The listing builds one solid part. Answer for the finished solid, in the listing's coordinates (mm). A direction names the side the tool comes from. Give positions to 0.01 mm unless a question says otherwise; leave off trailing zeros. Loops run counter-clockwise (first coordinate to the right, second up) from the corner with the lowest first, then second, coordinate; pieces in that order, holes last. Notation, with made-up numbers: M -18.5,14.5 L 7.5,14.5 A23 cw 7.5,53.5 Z; hole C 18.5,-29 d6. An arc over 180 degrees is marked long. Return JSON: item names as keys, results as strings.
from build123d import *

# Parameters (mm, degrees)
F0_W     = 45.36
F0_H     = 15
F0_R     = 1.85
F1_DEPTH = 8
F3_DEPTH = 25
F5_DEPTH = 100


with BuildPart() as f1:
    # F0 (on Top) → F1 (new body)
    with BuildSketch(Plane.XY):
        with BuildLine():
            ThreePointArc((27.5, -14), (17.600505, -9.899495), (13.5, 0))
            ThreePointArc((13.5, 0), (0, 13.5), (-13.5, 0))
            ThreePointArc((-13.5, 0), (-17.600505, -9.899495), (-27.5, -14))
            Line((-27.5, -14), (-50, -14))
            Line((-50, -14), (-50, -64))
            Line((-50, -64), (50, -64))
            Line((50, -64), (50, -14))
            Line((50, -14), (27.5, -14))
        make_face()
        with Locations((0, -29.65)):
            Rectangle(F0_W, F0_H, mode=Mode.SUBTRACT)
        with Locations((-8, 0)):
            Circle(F0_R, mode=Mode.SUBTRACT)
        with Locations((0, -8)):
            Circle(F0_R, mode=Mode.SUBTRACT)
        with Locations((8, 0)):
            Circle(F0_R, mode=Mode.SUBTRACT)
        with Locations((0, 8)):
            Circle(F0_R, mode=Mode.SUBTRACT)
    extrude(amount=F1_DEPTH)

    # F2 (on face) → F3 (join)
    with BuildSketch(Plane.XY.offset(8)):
        Polygon((-27.5, -14), (-50, -14), (-50, -64), (50, -64), (50, -14), (27.5, -14), (22.68, -14), (22.68, -22.15), (22.68, -37.15), (-22.68, -37.15), (-22.68, -22.15), (-22.68, -14), align=None)
    extrude(amount=F3_DEPTH)

    # F4 (on face) → F5 (cut, through all)
    with BuildSketch(Plane(origin=(-50, 0, 0), x_dir=(0, -1, 0), z_dir=(-1, 0, 0))):
        Polygon((24.292708, 33), (25.35, 8), (52.65, 8), (53.707292, 33), align=None)
    extrude(amount=-F5_DEPTH, mode=Mode.SUBTRACT)


solid = f1.part
(1) A tool of negligible diameter and unlimited length cuts with its end or side. For faces 1 (the flat face through (0, -37.15, 4)), 2 (the flat face through (-1, -42, 8)), 3 (the flat face through (50, -39, 5)), 4 (the flat face through (-37, -19, 33)), 5 (the flat face through (-22.68, -23, 16)), from which of +Z, -Z, +X, -X, +Y, -Y can it reach the whole face along a straight path? Write none if from no direction.
Values follow:
{"face 1": "+Z, -Z", "face 2": "+Z, +X, -X", "face 3": "+Z, -Z, +X, +Y, -Y", "face 4": "+Z, +X, -X, +Y, -Y", "face 5": "+Z"}
(2) The part is cut by section D-D (x = 31). Determine the outline of the cut face in (y, z), and give its area (3 significant figures).
Values follow:
{"outline": "M -64,0 L -14,0 L -14,33 L -24.29,33 L -25.35,8 L -52.65,8 L -53.71,33 L -64,33 Z", "area": "941 mm²"}
(3) Given pin 1 (18 mm diameter, centred on x = -11.5, y = -12, fed in from +Z); pin 2 (4 mm diameter, centred on x = 30.5, z = 29.5, fed in from +Y), each flat-ended and moving along its own axis, determine where each tip first touches the part or whether it passes through.
Values follow:
{"pin 1": "z = 8", "pin 2": "y = -14"}
(4) The part is cut by section B-B (x = 0). Determine the outline of the cut face in (y, z).
Values follow:
{"outline": "M -64,0 L -37.15,0 L -37.15,8 L -52.65,8 L -53.71,33 L -64,33 Z; M -22.15,0 L -9.85,0 L -9.85,8 L -22.15,8 Z; M -6.15,0 L 6.15,0 L 6.15,8 L -6.15,8 Z; M 9.85,0 L 13.5,0 L 13.5,8 L 9.85,8 Z"}
(5) The part is cut by section A-A (y = -27). Determine the outline of the cut face in (x, z), and give its area (3 significant figures).
Values follow:
{"outline": "M -50,0 L -22.68,0 L -22.68,8 L -50,8 Z; M 22.68,0 L 50,0 L 50,8 L 22.68,8 Z", "area": "437 mm²"}
(6) The part is cut by section C-C (z = 23). Determine the outline of the cut face in (x, y).
Values follow:
{"outline": "M -50,-64 L 50,-64 L 50,-53.28 L -50,-53.28 Z; M -50,-24.72 L -22.68,-24.72 L -22.68,-14 L -50,-14 Z; M 22.68,-24.72 L 50,-24.72 L 50,-14 L 22.68,-14 Z"}
(7) Straight lines are drawn through the part: line 1 along Y through (x, z) = (0, 2); line 2 along Y through (x, z) = (8, 3); line 3 along X through (y, z) = (-32.5, 2). For each, find the intervals that lie inside material, in ascending order.
Values follow:
{"line 1": "-64 to -37.15, -22.15 to -9.85, -6.15 to 6.15, 9.85 to 13.5", "line 2": "-64 to -37.15, -22.15 to -1.85, 1.85 to 10.87", "line 3": "-50 to -22.68, 22.68 to 50"}
(8) Determine the mould class of faces 6 (the flat face through (22.68, -23, 16)), 7 (the flat face through (37, -14, 16)), 8 (the cylindrical face through (6.15, 0.08, 3.94)), 9 (the flat face through (-1, -42, 0)) for opening direction Y: released by +Y, released by -Y, zero draft, split by the parting line, or undercut.
Values follow:
{"face 6": "undercut", "face 7": "released by +Y", "face 8": "undercut", "face 9": "zero draft"}
